from build123d import *

# Parameters (mm, degrees)
F0_W      = 120
F0_H      = 130
F1_DEPTH  = 10
F2_W      = 120
F2_H      = 10
F3_DEPTH  = 10
F4_W      = 14
F4_H      = 3
F5_DEPTH  = 25
F6_DEPTH  = 25
F7_R      = 2
F8_DEPTH  = 25
F9_W      = 14
F9_H      = 7
F10_DEPTH = 2
F11_W     = 80
F11_H     = 80
F12_DEPTH = 25


with BuildPart() as f1:
    # F0 (on Top) → F1 (new body)
    with BuildSketch(Plane.XY):
        with Locations((1.984598, 20.88183)):
            Rectangle(F0_W, F0_H)
    extrude(amount=F1_DEPTH)

    # F2 (on face) → F3 (join)
    with BuildSketch(Plane.XY.offset(10)):
        with Locations((1.984598, 80.88183)):
            Rectangle(F2_W, F2_H)
    extrude(amount=F3_DEPTH)

    # F4 (on face) → F5 (cut)
    with BuildSketch(Plane.XZ.offset(-75.88183)):
        with Locations((-36.015402, 11.5)):
            Rectangle(F4_W, F4_H)
    extrude(amount=-F5_DEPTH, mode=Mode.SUBTRACT)

    # F4 (on face) → F6 (cut)
    with BuildSketch(Plane.XZ.offset(-75.88183)):
        with Locations((39.984598, 11.5)):
            Rectangle(F4_W, F4_H)
    extrude(amount=-F6_DEPTH, mode=Mode.SUBTRACT)

    # F7 (on face) → F8 (cut)
    with BuildSketch(Plane.XY.offset(10)):
        with Locations((-48.015402, 65.88183)):
            Circle(F7_R)
        with Locations((51.984598, 65.88183)):
            Circle(F7_R)
        with Locations((51.984598, -34.11817)):
            Circle(F7_R)
        with Locations((-48.015402, -34.11817)):
            Circle(F7_R)
    extrude(amount=-F8_DEPTH, mode=Mode.SUBTRACT)

    # F9 (on face) → F10 (cut)
    with BuildSketch(Plane.XY.offset(10)):
        with Locations((-36.015402, -40.61817)):
            Rectangle(F9_W, F9_H)
        with Locations((39.984598, -40.61817)):
            Rectangle(F9_W, F9_H)
    extrude(amount=-F10_DEPTH, mode=Mode.SUBTRACT)

    # F11 (on face) → F12 (cut)
    with BuildSketch(Plane.XY.offset(10)):
        with Locations((1.984598, 15.88183)):
            Rectangle(F11_W, F11_H)
    extrude(amount=-F12_DEPTH, mode=Mode.SUBTRACT)


solid = f1.part
Check sheet for the modelled part. Datum: model origin and axes. Units: mm. A direction names the side the tool comes from. Coordinates: 2 decimals unless noted, no trailing zeros. Write each loop counter-clockwise with the first axis right and the second up, starting at its lowest first coordinate (ties: lowest second). Pieces come first, ordered by that corner, then holes.
Item 1: Cross-section at C-C on z = 5. Record the boundary of the cut face in (x, y), then the cut area to 3 significant figures.
Numbers:
outline: (-58.02, -44.12) - (61.98, -44.12) - (61.98, 85.88) - (-58.02, 85.88) - close; hole circle Ø4 at (-48.02, -34.12); hole circle Ø4 at (-48.02, 65.88); hole (-38.02, -24.12) - (41.98, -24.12) - (41.98, 55.88) - (-38.02, 55.88) - close; hole circle Ø4 at (51.98, -34.12); hole circle Ø4 at (51.98, 65.88)
area: 9,150 mm2
Item 2: Scan lines: probe 1 along X at (y, z) = (12, 9.75); probe 2 along Y at (x, z) = (-15, 1.25); probe 3 along Z at (x, y) = (-21, 71). Record each from-to range of solid material in increasing order.
Numbers:
probe 1: x = -58.02 to -38.02, 41.98 to 61.98
probe 2: y = -44.12 to -24.12, 55.88 to 85.88
probe 3: z = 0 to 10
Item 3: Mould release check, pull along Y, two halves, no side actions. Record for faces 5 (the face through (1, -24.118, 5)), 6 (the face through (1, 85.882, 10)), 7 (the face through (1, 81, 20)): released by +Y, released by -Y, zero draft, split by the parting line, or undercut.
Numbers:
face 5: undercut
face 6: released by +Y
face 7: zero draft
Item 4: Cross-section at D-D on x = -41.5. Record the boundary of the cut face in (y, z), then the cut area to 3 significant figures.
Numbers:
outline: (-44.12, 0) - (85.88, 0) - (85.88, 10) - (-37.12, 10) - (-37.12, 8) - (-44.12, 8) - close; (75.88, 13) - (85.88, 13) - (85.88, 20) - (75.88, 20) - close
area: 1,360 mm2
Item 5: Depth check by flat-ended pin: pin 1 Ø1 at (x, y) = (-10.5, 69.5) entering from +Z; pin 2 Ø1 at (x, z) = (39.5, 9) entering from -Y; pin 3 Ø11 at (x, z) = (28, 17) entering from -Y. Enter the tip coordinate at first touch or a pass-through.
Numbers:
pin 1: stops at z = 10
pin 2: stops at y = -37.12
pin 3: stops at y = 75.88
Item 6: Access from +Z, -Z, +X, -X, +Y, -Y to the whole of each face (thin tool, end or side, straight path). Record for faces 1 (the face through (-29.015, 81, 11)), 2 (the face through (41.985, 15, 5)), 3 (the face through (-36, -41, 8)), 4 (the face through (1, -44.118, 5)).
Numbers:
face 1: +Y, -Y
face 2: +Z, -Z
face 3: +Z, -Y
face 4: +Z, -Z, +X, -X, -Y
Item 7: Cross-section at A-A on x = -19. Record the boundary of the cut face in (y, z), then the cut area to 3 significant figures.
Numbers:
outline: (-44.12, 0) - (-24.12, 0) - (-24.12, 10) - (-44.12, 10) - close; (55.88, 0) - (85.88, 0) - (85.88, 20) - (75.88, 20) - (75.88, 10) - (55.88, 10) - close
area: 600 mm2
Item 8: Cross-section at B-B on y = 42.5. Record the boundary of the cut face in (x, z), then the cut area to 3 significant figures.
Numbers:
outline: (-58.02, 0) - (-38.02, 0) - (-38.02, 10) - (-58.02, 10) - close; (41.98, 0) - (61.98, 0) - (61.98, 10) - (41.98, 10) - close
area: 400 mm2
